from build123d import *

# Parameters (mm, degrees)
SKETCH_1_R          = 35
SKETCH_1_R_2        = 22.5
SKETCH_1_R_3        = 2.25
EXTRUDE_1_DEPTH     = 4
EXTRUDE_2_DEPTH     = 4
SKETCH_3_W          = 30
SKETCH_3_H          = 10
EXTRUDE_3_DEPTH     = 34
EXTRUDE_4_DEPTH     = 4
SKETCH_5_R          = 9.5
EXTRUDE_5_DEPTH     = 52.5
SKETCH_6_W          = 29
SKETCH_6_H          = 29
SKETCH_6_W_2        = 15
CUT_EXTRUDE_1_DEPTH = 28
CUT_EXTRUDE_2_REACH = 149.879
SKETCH_7_R          = 11
FILLET_1_R          = 15
FILLET_3_R          = 5
CHAMFER_1_SIZE      = 2.5
CHAMFER_2_SIZE      = 10


with BuildPart() as part:
    # 草图1 → 凸台-拉伸1 (new body)
    with BuildSketch(Plane(origin=(0, 0, 0), x_dir=(1, 0, 0), z_dir=(0, 1, 0))):
        with Locations(Location((0, 0, 0), (0, 0, 270))):
            Circle(SKETCH_1_R)
        with Locations(Location((0, 0, 0), (0, 0, 270))):
            Circle(SKETCH_1_R_2, mode=Mode.SUBTRACT)
        with Locations(Location((-9.918584156, 27.251086003, 0), (0, 0, 270))):
            Circle(SKETCH_1_R_3, mode=Mode.SUBTRACT)
        with Locations(Location((9.918584156, 27.251086003, 0), (0, 0, 270))):
            Circle(SKETCH_1_R_3, mode=Mode.SUBTRACT)
        with Locations(Location((28.559424837, -5.035797152, 0), (0, 0, 270))):
            Circle(SKETCH_1_R_3, mode=Mode.SUBTRACT)
        with Locations(Location((18.640840681, -22.21528885, 0), (0, 0, 270))):
            Circle(SKETCH_1_R_3, mode=Mode.SUBTRACT)
        with Locations(Location((-18.640840681, -22.21528885, 0), (0, 0, 270))):
            Circle(SKETCH_1_R_3, mode=Mode.SUBTRACT)
        with Locations(Location((-28.559424837, -5.035797152, 0), (0, 0, 270))):
            Circle(SKETCH_1_R_3, mode=Mode.SUBTRACT)
    extrude(amount=EXTRUDE_1_DEPTH)

    # 草图2 → 凸台-拉伸2 (add)
    with BuildSketch(Plane(origin=(0, 0, 0), x_dir=(1, 0, 0), z_dir=(0, 1, 0))):
        with BuildLine():
            Line((15, -42.426406871), (15, -31.622776602))
            ThreePointArc((15, -31.622776602), (0, -35), (-15, -31.622776602))
            Line((-15, -31.622776602), (-15, -42.426406871))
            ThreePointArc((-15, -42.426406871), (0, -45), (15, -42.426406871))
        make_face()
    extrude_2 = extrude(amount=EXTRUDE_2_DEPTH)

    # 草图3 → 凸台-拉伸3 (add)
    with BuildSketch(Plane(origin=(0, 0, 0), x_dir=(1, 0, 0), z_dir=(0, 1, 0))):
        with Locations((0, -40)):
            Rectangle(SKETCH_3_W, SKETCH_3_H)
    extrude_3 = extrude(amount=EXTRUDE_3_DEPTH)

    # 镜向1: 凸台-拉伸2, 凸台-拉伸3 across plane
    add(extrude_2.mirror(Plane.XY))
    add(extrude_3.mirror(Plane.XY))

    # 草图4 → 凸台-拉伸4 (add)
    with BuildSketch(Plane(origin=(0, 0, 0), x_dir=(1, 0, 0), z_dir=(0, 1, 0))):
        with BuildLine():
            Line((-52.5, 89), (52.5, 89))
            Line((52.5, 89), (52.5, 30.310889132))
            Line((52.5, 30.310889132), (30.310889132, 17.5))
            ThreePointArc((30.310889132, 17.5), (0, 35), (-30.310889132, 17.5))
            Line((-30.310889132, 17.5), (-52.5, 30.310889132))
            Line((-52.5, 30.310889132), (-52.5, 89))
        make_face()
    extrude(amount=EXTRUDE_4_DEPTH)

    # 草图5 → 凸台-拉伸5 (add, symmetric)
    with BuildSketch(Plane(origin=(0, 0, 0), x_dir=(0, 0, -1), z_dir=(1, 0, 0))):
        with BuildLine():
            Line((89, 4), (61, 4))
            Line((61, 4), (61, 19))
            ThreePointArc((61, 19), (75, 33), (89, 19))
            Line((89, 19), (89, 4))
        make_face()
        with Locations((75, 19)):
            Circle(SKETCH_5_R, mode=Mode.SUBTRACT)
    extrude(amount=EXTRUDE_5_DEPTH, both=True)

    # 草图6 → 切除-拉伸1 (cut)
    with BuildSketch(Plane(origin=(0, 0, -89), x_dir=(-1, 0, 0), z_dir=(0, 0, -1))):
        with Locations((-30, 18.5)):
            Rectangle(SKETCH_6_W, SKETCH_6_H)
        with Locations((0, 18.5)):
            Rectangle(SKETCH_6_W_2, SKETCH_6_H)
        with Locations((30, 18.5)):
            Rectangle(SKETCH_6_W, SKETCH_6_H)
    extrude(amount=-CUT_EXTRUDE_1_DEPTH, mode=Mode.SUBTRACT)

    # 切除-拉伸2: up to this face of the body (flat: up to its plane)
    cut_extrude_2_end = Plane(part.part.faces().sort_by_distance((0, 19, -45))[0])
    # 草图7 → 切除-拉伸2 (cut, up to the picked face)
    with BuildSketch(Plane.XY.offset(45), mode=Mode.PRIVATE) as cut_extrude_2_sk1:
        with Locations((0, 19)):
            Circle(SKETCH_7_R)
    cut_extrude_2_tool1 = split(extrude(cut_extrude_2_sk1.sketch, amount=-CUT_EXTRUDE_2_REACH, mode=Mode.PRIVATE), bisect_by=cut_extrude_2_end, keep=Keep.BOTH, mode=Mode.PRIVATE)
    add(cut_extrude_2_tool1.solids().sort_by(Axis((0, 19, 45), (0, 0, -1)))[0], mode=Mode.SUBTRACT)

    # 圆角1
    fillet_1_edges = [part.edges().sort_by_distance(p)[0] for p in [
        (15, 34, -40),
        (-15, 34, -40),
        (-15, 34, 40),
        (15, 34, 40),
    ]]
    fillet(fillet_1_edges, radius=FILLET_1_R - 0.0001)  # a hair under: the kernel refuses the full size

    # 圆角3
    fillet_3_edges = [part.edges().sort_by_distance(p)[0] for p in [
        (-30.310889132, 2, -17.5),
        (30.310889132, 2, -17.5),
        (52.5, 2, -30.310889132),
        (-52.5, 2, -30.310889132),
        (15, 2, 31.622776602),
        (-15, 2, 31.622776602),
    ]]
    fillet(fillet_3_edges, radius=FILLET_3_R)

    # 倒角1
    chamfer_1_edges = [part.edges().sort_by_distance(p)[0] for p in [
        (-9.918584156, 4, -29.501086003),
        (28.559424837, 4, 2.785797152),
        (18.640840681, 4, 19.96528885),
        (-18.640840681, 4, 19.96528885),
        (-28.559424837, 4, 2.785797152),
        (9.918584156, 4, -29.501086003),
    ]]
    chamfer(chamfer_1_edges, length=CHAMFER_1_SIZE)

    # 倒角2
    chamfer_2_edges = [part.edges().sort_by_distance(p)[0] for p in [
        (48.5, 4, -61),
        (11.5, 4, -61),
        (-11.5, 4, -61),
        (-48.5, 4, -61),
    ]]
    chamfer(chamfer_2_edges, length=CHAMFER_2_SIZE)


solid = part.part
Here's how the part is built. I have some questions about the finished solid (model axes, mm). A direction names the side the tool comes from. Give positions to 0.01 mm unless a question says otherwise; leave off trailing zeros. Write each loop counter-clockwise with the first axis right and the second up, starting at its lowest first coordinate (ties: lowest second). Pieces come first, ordered by that corner, then holes. Notation, with made-up numbers: (57, 61) -> (92, 61) arc R19 cw to (92, 71) -> close; hole circle Ø3 at (-24.75, 0). An arc over 180 degrees is marked (long way). Use one line per item in the form item = value. Start each with the question number.
1. Thinking about a two-plate mould opening in Z: for faces 4 (the face through (12, 16, -61)), 5 (the face through (-10.72, 29.49, 39.93)), 6 (the face through (-16.41, 0.74, 21.92)), 7 (the face through (-48, 33, -75)), which applies, +Z half, -Z half, draft (parallel to the pull), parting line (faces both ways), or undercut?
2. Imagine slicing it at A-A on y = 6.5. List the corners of the cut face in (x, z) for me, plus the area to 3 significant figures.
3. Imagine slicing it at B-B on z = -75. State how many separate pieces and enclosed holes the cut face has, plus the area to 3 significant figures.
4. Imagine slicing it at D-D on z = -4. List the corners of the cut face in (x, y) for me.
5. Imagine slicing it at C-C on z = -18. List the corners of the cut face in (x, y) for me.
6. If I drill on L1, parallel to Z at x = -13.5, y = 19; L2, parallel to Y at x = 0.5, z = -43.5; L3, parallel to X at y = 1, z = 0, over which ranges is the centre line in solid material (lowest first)?
7. On a 3-axis mill with a long thin cutter (end or side, diameter ignored), from which of +Z, -Z, +X, -X, +Y, -Y can I reach the whole of each face in a straight line? I mean faces 1 (the face through (10.72, 29.49, 39.93)), 2 (the face through (6, 9, -45)), 3 (the face through (12.15, 0.74, -27.54)). Say none if no direction works.
8. Will these pins go through, and if not, where does the flat tip stop? pin 1 Ø8.5 at (y, z) = (8.5, 41) entering from -X; pin 2 Ø1 at (x, y) = (-1.5, 7.5) entering from -Z; pin 3 Ø5 at (x, z) = (9.92, -27.25) entering from +Y.
Entries:
q1.face_4 = undercut
q1.face_5 = draft
q1.face_6 = undercut
q1.face_7 = parting line
q2.outline = (-52.5, -89) -> (-44.5, -89) -> (-44.5, -53.5) -> (-52.5, -53.5) -> close; (-15.5, -89) -> (-7.5, -89) -> (-7.5, -53.5) -> (-15.5, -53.5) -> close; (-15, -45) -> (15, -45) -> (15, -35) -> (-15, -35) -> close; (-15, 35) -> (15, 35) -> (15, 45) -> (-15, 45) -> close; (7.5, -89) -> (15.5, -89) -> (15.5, -53.5) -> (7.5, -53.5) -> close; (44.5, -89) -> (52.5, -89) -> (52.5, -53.5) -> (44.5, -53.5) -> close
q2.area = 1,740 mm²
q3.separate_pieces = 5
q3.enclosed_holes = 0
q3.area = 740 mm²
q4.outline = (-34.77, 0) -> (-22.14, 0) -> (-22.14, 4) -> (-34.77, 4) -> close; (22.14, 0) -> (34.77, 0) -> (34.77, 4) -> (22.14, 4) -> close
q5.outline = (-32.53, 0) -> (-13.5, 0) -> (-13.5, 4) -> (-32.53, 4) -> close; (13.5, 0) -> (32.53, 0) -> (32.53, 4) -> (13.5, 4) -> close
q6.L1 = -89 to -84.5, -65.5 to -61, -45 to -35, 35 to 45
q6.L2 = 0 to 8.01, 29.99 to 33.99
q6.L3 = -35 to -22.5, 22.5 to 35
q7.face_1 = +Z, +X, +Y
q7.face_2 = +X, -X, +Y
q7.face_3 = +Y, -Y
q8.pin_1 = -15
q8.pin_2 = -45
q8.pin_3 = 1.75
